Work out the finished part from the listing and answer in its coordinate system (mm). Give positions to 0.01 mm unless a question says otherwise; leave off trailing zeros. Loops run counter-clockwise (first coordinate to the right, second up) from the corner with the lowest first, then second, coordinate; pieces in that order, holes last.
```python
from build123d import *

# Parameters (mm, degrees)
BOSS_EXTRUDE1_DEPTH = 2


with BuildPart() as part:
    # Sketch3 → Boss-Extrude1 (new body)
    with BuildSketch(Plane(origin=(0, 0, 0), x_dir=(1, 0, 0), z_dir=(0, 1, 0))):
        with BuildLine():
            Line((158, 22.5), (158, -81))
            ThreePointArc((158, -81), (157.121320344, -83.121320344), (155, -84))
            Line((155, -84), (53.050466482, -84))
            ThreePointArc((53.050466482, -84), (8.545143105, -89.838724048), (-32.948056713, -106.959730921))
            ThreePointArc((-32.948056713, -106.959730921), (-35.225053269, -107.255305993), (-37.044136112, -105.854229426))
            Line((-37.044136112, -105.854229426), (-70.68813753, -47.336444363))
            ThreePointArc((-70.68813753, -47.336444363), (-70.983712602, -45.059447807), (-69.582636034, -43.240364964))
            ThreePointArc((-69.582636034, -43.240364964), (-32.385273168, -15.689281312), (-2.499253861, 19.659436693))
            ThreePointArc((-2.499253861, 19.659436693), (-1.418042651, 20.643701012), (0, 21))
            ThreePointArc((0, 21), (12.831153008, 22.8704149), (24.594386694, 28.325987526))
            ThreePointArc((24.594386694, 28.325987526), (35.310753338, 33.296042365), (47, 35))
            ThreePointArc((47, 35), (65.898115208, 34.170434491), (84.650849693, 31.688119703))
            ThreePointArc((84.650849693, 31.688119703), (119.689605729, 27.050010933), (155, 25.5))
            ThreePointArc((155, 25.5), (157.121320344, 24.621320344), (158, 22.5))
        make_face()
    extrude(amount=-BOSS_EXTRUDE1_DEPTH)


solid = part.part
```
Q1. Section C-C on z = 31 is taken. Give the vertices of the cut face in (x, y).
Q2. Section B-B on x = 133 is taken. Give the vertices of the cut face in (y, z), plus the area to 3 significant figures.
Q3. Given pin 1 (1 mm diameter, centred on x = 10.5, y = -0.5, fed in from +Z), flat-ended and moving along its own axis, determine where the tip first touches the part or whether it passes through.
Q4. Consider line 1 along X through (y, z) = (-0.4, 38.5); line 2 along Z through (x, y) = (98, -1.15); line 3 along X through (y, z) = (-1.7, 76). Determine where each line is inside the solid, lowest interval first.
Q5. Section A-A on y = -0.85 is taken. Give the vertices of the cut face in (x, z).
Check result:
1. outline: (-50.81, -2) - (158, -2) - (158, 0) - (-50.81, 0) - close
2. outline: (-2, -26.1) - (0, -26.1) - (0, 84) - (-2, 84) - close
2. area: 220 mm2
3. pin 1: stops at z = 89.46
4. line 1: x = -61.76 to 158
4. line 2: z = -29.55 to 84
4. line 3: x = -54.21 to 158
5. outline: (-70.69, 47.34) arc R3 ccw to (-69.58, 43.24) arc R200.46 cw to (-2.5, -19.66) arc R3 ccw to (0, -21) arc R44.95 cw to (24.59, -28.33) arc R40.95 ccw to (47, -35) arc R215.67 ccw to (84.65, -31.69) arc R402.97 cw to (155, -25.5) arc R3 ccw to (158, -22.5) - (158, 81) arc R3 ccw to (155, 84) - (53.05, 84) arc R172.54 cw to (-32.95, 106.96) arc R3 ccw to (-37.04, 105.85) - close
